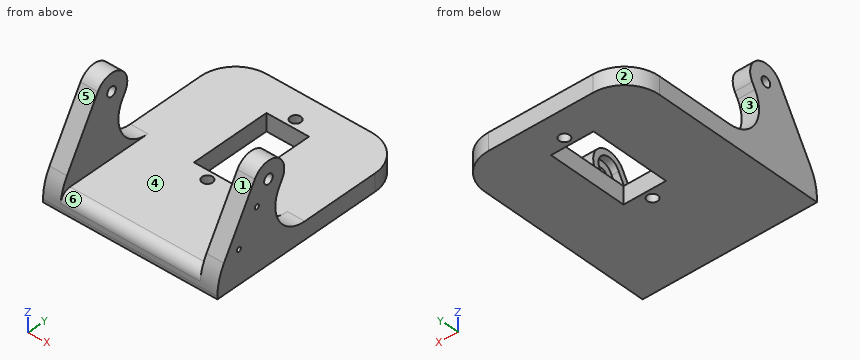
from build123d import *

# Parameters (mm, degrees)
ESQUISSE1_W                  = 50
ESQUISSE1_H                  = 60
BOSS_EXTRU_1_DEPTH           = 5
ESQUISSE2_W                  = 12.2
ESQUISSE2_H                  = 23
ENL_V_MAT_EXTRU_1_DEPTH      = 40.37003937
ESQUISSE3_R                  = 1.5
ENL_V_MAT_EXTRU_2_DEPTH      = 40.37003937
BOSS_EXTRU_2_DEPTH           = 5
CONG_1_RADIUS                = 5
CONG_1_LENGTH                = 5
CONG_2_R                     = 9.35
ENL_V_MAT_EXTRU_3_DEPTH      = 2
ESQUISSE6_R                  = 0.65
ESQUISSE6_R_2                = 1.375
ENL_V_MAT_EXTRU_4_DEPTH      = 61.942279509
CONG_1_OF_SYM_TRIE1_2_RADIUS = 5
CONG_1_OF_SYM_TRIE1_2_LENGTH = 5
CONG_2_OF_SYM_TRIE1_R        = 9.35
ESQUISSE7_R                  = 1.375
ENL_V_MAT_EXTRU_5_DEPTH      = 65.722186549
CONG_3_R                     = 15.5
CONG_4_R                     = 3
CONG_5_R                     = 10


with BuildPart() as part:
    # Esquisse1 → Boss.-Extru.1 (new body)
    with BuildSketch(Plane.XY):
        Rectangle(ESQUISSE1_W, ESQUISSE1_H)
    extrude(amount=BOSS_EXTRU_1_DEPTH)

    # Esquisse2 → Enlèv. mat.-Extru.1 (cut, through all)
    with BuildSketch(Plane.XY.offset(5)):
        with Locations((0, 8.5)):
            Rectangle(ESQUISSE2_W, ESQUISSE2_H)
    extrude(amount=-ENL_V_MAT_EXTRU_1_DEPTH, mode=Mode.SUBTRACT)

    # Esquisse3 → Enlèv. mat.-Extru.2 (cut, through all)
    with BuildSketch(Plane(origin=(0, 0, 0), x_dir=(-1, 0, 0), z_dir=(0, 0, -1))):
        with Locations((0, -5.5)):
            Circle(ESQUISSE3_R)
        with Locations((0, 22.5)):
            Circle(ESQUISSE3_R)
    extrude(amount=-ENL_V_MAT_EXTRU_2_DEPTH, mode=Mode.SUBTRACT)

    # Esquisse4 → Boss.-Extru.2 (add)
    with BuildSketch(Plane(origin=(25, 0, 0), x_dir=(0, 0, -1), z_dir=(1, 0, 0))):
        Polygon((-5, -30), (-29.918584287, -15.613248654), (-24.918584287, -6.952994616), (-5, -18.452994616), align=None)
    boss_extru_2 = extrude(amount=-BOSS_EXTRU_2_DEPTH)

    # Congé1: full round fillet: the end face becomes a half cylinder, R = half its width
    cong_1_face = Plane((22.5, -11.283121635, 27.418584287), x_dir=(1, 0, 0), z_dir=(0, 0.5, 0.866025403784))  # on the end face: x along it, z out of the body
    cong_1_slab = cong_1_face.offset(-CONG_1_RADIUS / 2) * Box(CONG_1_LENGTH, 2 * CONG_1_RADIUS, CONG_1_RADIUS, mode=Mode.PRIVATE)  # the body's end, R deep
    cong_1_round = Plane((22.5, -13.783121635, 23.088457268), x_dir=(0, 0.5, 0.866025403784), z_dir=(1, 0, 0)) * Cylinder(CONG_1_RADIUS, CONG_1_LENGTH, mode=Mode.PRIVATE)  # its axis R under the face
    add(cong_1_slab - cong_1_round, mode=Mode.SUBTRACT)

    # Congé2
    cong_2_edges = [part.edges().sort_by_distance(p)[0] for p in [
        (22.5, -18.452994616, 5),
    ]]
    fillet(cong_2_edges, radius=CONG_2_R)

    # Esquisse5 → Enlèv. mat.-Extru.3 (cut)
    with BuildSketch(Plane.ZY.offset(-20)):
        with BuildLine():
            Line((10.742191848, -24.653283165), (24.350818961, -16.858928401))
            ThreePointArc((24.350818961, -16.858928401), (25.938192754, -12.070476908), (20.964861107, -11.224902792))
            Line((20.964861107, -11.224902792), (8.56647232, -21.51689595))
            ThreePointArc((8.56647232, -21.51689595), (8.216016866, -24.082852363), (10.742191848, -24.653283165))
        make_face()
    extrude(amount=-ENL_V_MAT_EXTRU_3_DEPTH, mode=Mode.SUBTRACT)

    # Esquisse6 → Enlèv. mat.-Extru.4 (cut, through all)
    with BuildSketch(Plane.ZY.offset(-20)):
        with Locations((9.522873524, -23.175934722)):
            Circle(ESQUISSE6_R)
        with Locations((17.74443943, -17.48332073)):
            Circle(ESQUISSE6_R)
        with Locations((23.088457268, -13.783121635)):
            Circle(ESQUISSE6_R_2)
    extrude(amount=-ENL_V_MAT_EXTRU_4_DEPTH, mode=Mode.SUBTRACT)

    # Symétrie1: Boss.-Extru.2 across plane
    add(boss_extru_2.mirror(Plane(origin=(0, 0, 0), x_dir=(0, 0, 1), z_dir=(1, 0, 0))))

    # Congé1 of Sym_trie1 2: full round fillet: the end face becomes a half cylinder, R = half its width
    cong_1_of_sym_trie1_2_face = Plane((-22.5, -11.283121635, 27.418584287), x_dir=(-1, 0, 0), z_dir=(0, 0.5, 0.866025403784))  # on the end face: x along it, z out of the body
    cong_1_of_sym_trie1_2_slab = cong_1_of_sym_trie1_2_face.offset(-CONG_1_OF_SYM_TRIE1_2_RADIUS / 2) * Box(CONG_1_OF_SYM_TRIE1_2_LENGTH, 2 * CONG_1_OF_SYM_TRIE1_2_RADIUS, CONG_1_OF_SYM_TRIE1_2_RADIUS, mode=Mode.PRIVATE)  # the body's end, R deep
    cong_1_of_sym_trie1_2_round = Plane((-22.5, -13.783121635, 23.088457268), x_dir=(0, 0.5, 0.866025403784), z_dir=(-1, 0, 0)) * Cylinder(CONG_1_OF_SYM_TRIE1_2_RADIUS, CONG_1_OF_SYM_TRIE1_2_LENGTH, mode=Mode.PRIVATE)  # its axis R under the face
    add(cong_1_of_sym_trie1_2_slab - cong_1_of_sym_trie1_2_round, mode=Mode.SUBTRACT)

    # Congé2 of Symétrie1
    cong_2_of_sym_trie1_edges = [part.edges().sort_by_distance(p)[0] for p in [
        (-22.5, -18.452994616, 5),
    ]]
    fillet(cong_2_of_sym_trie1_edges, radius=CONG_2_OF_SYM_TRIE1_R)

    # Esquisse7 → Enlèv. mat.-Extru.5 (cut, through all)
    with BuildSketch(Plane.ZY.offset(25)):
        with Locations((23.088457268, -13.783121635)):
            Circle(ESQUISSE7_R)
    extrude(amount=-ENL_V_MAT_EXTRU_5_DEPTH, mode=Mode.SUBTRACT)

    # Congé3
    # the kernel refuses this fillet: 15.5 mm, written as the material it takes off along each edge
    with BuildSketch(Plane(origin=(4.919274896, -30, 5), x_dir=(0, 0, -1), z_dir=(-1, 0, 0)), Plane(origin=(49.919274896, -30, 5), x_dir=(0, 0, -1), z_dir=(-1, 0, 0))) as cong_3_piece_1:
        with BuildLine():
            CenterArc((CONG_3_R * 0.267949192431, -CONG_3_R), CONG_3_R, 90, 30)
            Line((-CONG_3_R * 0.232050807569, -CONG_3_R * 0.133974596216), (-CONG_3_R * 0.242050807569, -CONG_3_R * 0.11665408814))
            Line((-CONG_3_R * 0.242050807569, -CONG_3_R * 0.11665408814), (-CONG_3_R * 0.00535898384862, CONG_3_R * 0.02))
            Line((-CONG_3_R * 0.00535898384862, CONG_3_R * 0.02), (CONG_3_R * 0.267949192431, CONG_3_R * 0.02))
            Line((CONG_3_R * 0.267949192431, CONG_3_R * 0.02), (CONG_3_R * 0.267949192431, 0))
        make_face()
    extrude(amount=54.838549792, mode=Mode.SUBTRACT)

    # Congé4
    cong_4_edges = [part.edges().sort_by_distance(p)[0] for p in [
        (0, -29.433212182, 5),
    ]]
    fillet(cong_4_edges, radius=CONG_4_R)

    # Congé5
    cong_5_edges = [part.edges().sort_by_distance(p)[0] for p in [
        (-25, 30, 2.5),
        (25, 30, 2.5),
    ]]
    fillet(cong_5_edges, radius=CONG_5_R)


solid = part.part
Work out the finished part from the listing and answer in its coordinate system (mm). Face numbers are marked on the shaded views. A direction names the side the tool comes from. Round coordinates to 2 decimals unless told otherwise and drop trailing zeros. Write each loop counter-clockwise with the first axis right and the second up, starting at its lowest first coordinate (ties: lowest second). Pieces come first, ordered by that corner, then holes. Notation, with made-up numbers: (-30, 47.25) -> (-18, 47.25) arc R20 ccw to (-18, 55.25) -> close; hole circle Ø2 at (58.5, 50). An arc over 180 degrees is marked (long way). Answer as CSV lines item,"result". Start each with the question number.
(1) The part is cut by section A-A, the plane x = 0. Give the vertices of the cut face in (y, z), then the cut area to 3 significant figures.
(2) The part is cut by section B-B, the plane z = 15.5. Give the vertices of the cut face in (x, y), then the cut area to 3 significant figures.
(3) The part is cut by section D-D, the plane x = 13.5. Give the vertices of the cut face in (y, z), then the cut area to 3 significant figures.
(4) Find the intervals of material crossed by probe 1 along X at (y, z) = (-10, 21.5); probe 2 along X at (y, z) = (-23, 8.5); probe 3 along Y at (x, z) = (0, 2.9), in increasing order.
(5) Each of these flat-tipped pins is pushed along its axis until it touches: pin 1 (15 mm diameter, centred on x = 10, y = -7, fed in from +Z); pin 2 (0.8 mm diameter, centred on y = -17.48, z = 17.74, fed in from +X). Where does it stop, or does it pass through?
(6) The part is cut by section C-C, the plane y = -1. Give the vertices of the cut face in (x, z).
(7) A tool of negligible diameter and unlimited length cuts with its end or side. For the marked faces 4, 5 and 6, from which of +Z, -Z, +X, -X, +Y, -Y can it reach the whole face along a straight path? Write none if from no direction.
(8) The mould has two halves that part along Z. Classify the marked faces 1, 2 and 3: +Z half, -Z half, draft (parallel to the pull), parting line (faces both ways), or undercut.
Output values:
1,outline,"(-30, 0) -> (-7, 0) -> (-7, 5) -> (-26.95, 5) arc R3 ccw to (-29.93, 2.28) arc R15.5 ccw to (-30, 0.85) -> close; (-4, 0) -> (-3, 0) -> (-3, 5) -> (-4, 5) -> close; (20, 0) -> (21, 0) -> (21, 5) -> (20, 5) -> close; (24, 0) -> (30, 0) -> (30, 5) -> (24, 5) -> close"
1,area,"153 mm²"
2,outline,"(-25, -23.94) -> (-20, -23.94) -> (-20, -11.54) -> (-25, -11.54) -> close; (20, -23.94) -> (25, -23.94) -> (25, -11.54) -> (20, -11.54) -> (20, -15.76) -> (22, -15.76) -> (22, -21.93) -> (20, -21.93) -> close"
2,area,"112 mm²"
3,outline,"(-30, 0) -> (30, 0) -> (30, 5) -> (-26.95, 5) arc R3 ccw to (-29.93, 2.28) arc R15.5 ccw to (-30, 0.85) -> close"
3,area,"298 mm²"
4,probe 1,"x = -25 to -20, 20 to 25"
4,probe 2,"x = -25 to -20, 22 to 25"
4,probe 3,"y = -29.81 to -7, -4 to -3, 20 to 21, 24 to 30"
5,pin 1,"stops at z = 5"
5,pin 2,"stops at x = -20"
6,outline,"(-25, 0) -> (-6.1, 0) -> (-6.1, 5) -> (-25, 5) -> close; (6.1, 0) -> (25, 0) -> (25, 5) -> (6.1, 5) -> close"
7,face 4,"+Z, +Y"
7,face 5,"+Z, +X, -X, -Y"
7,face 6,"+Z, -Y"
8,face 1,"+Z half"
8,face 2,"draft"
8,face 3,"undercut"
